from build123d import *

# Parameters (mm, degrees)
F0_W      = 38.3
F0_H      = 50.3
F0_W_2    = 28.3
F0_H_2    = 40.3
F4_DEPTH  = 4
F5_DEPTH  = 3
F5_FACE_W = 38.3
F5_FACE_H = 50.3
F7_DEPTH  = 35
F9_DEPTH  = 8
F10_R     = 5
F11_R     = 5


# Not quite as in the source:
# - the arcs of a loft's sections are written as splines that run evenly, so that the points pair up as in the source's solid


with BuildPart() as f4:
    # F0 (on Top) → F4 (new body)
    with BuildSketch(Plane.XY):
        Rectangle(F0_W, F0_H)
        Rectangle(F0_W_2, F0_H_2, mode=Mode.SUBTRACT)
    extrude(amount=-F4_DEPTH)

    # F0 (on Top) → F5 (join)
    with BuildSketch(Plane.XY):
        Rectangle(F0_W, F0_H)
        Rectangle(F0_W_2, F0_H_2, mode=Mode.SUBTRACT)
        Rectangle(F0_W_2, F0_H_2)
    extrude(amount=F5_DEPTH)

    # F5_face (on face) → F6 section 0
    with BuildSketch(Plane.XY.offset(3)):
        Rectangle(F5_FACE_W, F5_FACE_H)
    # F2 (on offset) → F6 section 1
    with BuildSketch(Plane.XY.offset(10)):
        with BuildLine():
            add(Edge.make_bspline(
                [(5.1493417049, 6.762712474), (4.2641047121, 7.436759727), (3.2451924408, 7.934526467), (1.09359433, 8.5024723272), (-0.0382449475, 8.5724279849), (-2.2434058754, 8.2737605906), (-3.3158598892, 7.9052550514), (-5.2388678728, 6.785443806), (-6.0886652211, 6.0345786977), (-6.762712474, 5.1493417049)],
                knots=[0, 0, 0, 0, 0.25, 0.25, 0.5, 0.5, 0.75, 0.75, 1, 1, 1, 1], degree=3))
            add(Edge.make_bspline(
                [(-6.762712474, 5.1493417049), (-7.436759727, 4.2641047121), (-7.934526467, 3.2451924408), (-8.5024723272, 1.09359433), (-8.5724279849, -0.0382449475), (-8.2737605906, -2.2434058754), (-7.9052550514, -3.3158598892), (-6.785443806, -5.2388678728), (-6.0345786977, -6.0886652211), (-5.1493417049, -6.762712474)],
                knots=[0, 0, 0, 0, 0.25, 0.25, 0.5, 0.5, 0.75, 0.75, 1, 1, 1, 1], degree=3))
            add(Edge.make_bspline(
                [(-5.1493417049, -6.762712474), (-4.2641047121, -7.436759727), (-3.2451924408, -7.934526467), (-1.09359433, -8.5024723272), (0.0382449475, -8.5724279849), (2.2434058754, -8.2737605906), (3.3158598892, -7.9052550514), (5.2388678728, -6.785443806), (6.0886652211, -6.0345786977), (6.762712474, -5.1493417049)],
                knots=[0, 0, 0, 0, 0.25, 0.25, 0.5, 0.5, 0.75, 0.75, 1, 1, 1, 1], degree=3))
            add(Edge.make_bspline(
                [(6.762712474, -5.1493417049), (7.436759727, -4.2641047121), (7.934526467, -3.2451924408), (8.5024723272, -1.09359433), (8.5724279849, 0.0382449475), (8.2737605906, 2.2434058754), (7.9052550514, 3.3158598892), (6.785443806, 5.2388678728), (6.0345786977, 6.0886652211), (5.1493417049, 6.762712474)],
                knots=[0, 0, 0, 0, 0.25, 0.25, 0.5, 0.5, 0.75, 0.75, 1, 1, 1, 1], degree=3))
        make_face()
    loft(ruled=True)

    # F7 (add): a face of the model
    f7_faces = [f4.faces().sort_by_distance(p)[0] for p in [
        (0, 0, 10),
    ]]
    extrude(f7_faces, amount=F7_DEPTH)

    # F3 (on Front) → F8 (revolve)
    with BuildSketch(Plane.XZ):
        with BuildLine():
            Line((0, 30.5), (0, 65.5))
            ThreePointArc((0, 65.5), (-12.3743686708, 60.3743686708), (-17.5, 48))
            Line((-17.5, 48), (0, 30.5))
        make_face()
        with BuildLine():
            ThreePointArc((-17.5, 48), (-12.3743686708, 60.3743686708), (0, 65.5))
            Line((0, 65.5), (-17.5, 65.5))
            Line((-17.5, 65.5), (-17.5, 48))
        make_face()
    revolve(axis=Axis((0, 0, 48), (0, 0, -1)))

    # F9 (cut): a face of the model
    f9_faces = [f4.faces().sort_by_distance(p)[0] for p in [
        (0, 0, 65.5),
    ]]
    extrude(f9_faces, amount=-F9_DEPTH, mode=Mode.SUBTRACT)

    # F10
    f10_edges = [f4.edges().sort_by_distance(p)[0] for p in [
        (17.5, 0, 57.5),
        (17.5, 0, 48),
    ]]
    fillet(f10_edges, radius=F10_R)

    # F11
    f11_edges = [f4.edges().sort_by_distance(p)[0] for p in [
        (-19.15, -25.15, -0.5),
        (-19.15, 25.15, -0.5),
        (19.15, 25.15, -0.5),
        (19.15, -25.15, -0.5),
    ]]
    fillet(f11_edges, radius=F11_R)


solid = f4.part
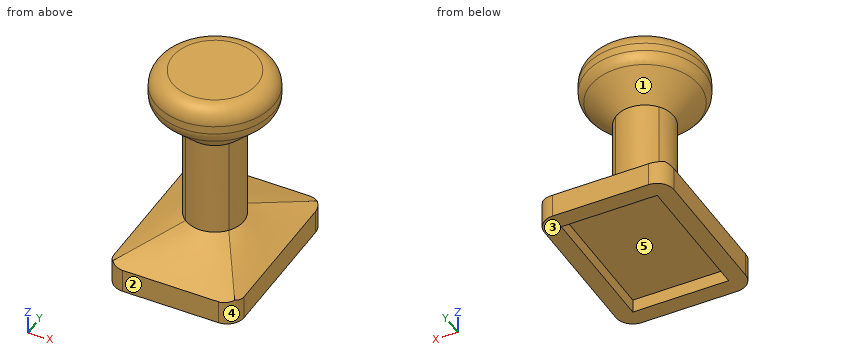
Check sheet for the modelled part. Datum: model origin and axes. Units: mm. Face numbers are marked on the shaded views. A direction names the side the tool comes from. Round coordinates to 2 decimals unless told otherwise and drop trailing zeros. Order: outer loops, then holes, each group sorted by start corner. A loop starts at its lowest first (then second) coordinate and runs counter-clockwise, first axis right, second up.
(1) Scan lines: probe 1 along Y at (x, z) = (-8.5, -0.5); probe 2 along Z at (x, y) = (6.5, 12.5); probe 3 along Z at (x, y) = (9, 14). Record each from-to range of solid material in increasing order.
(2) Go/stop test with flat-tipped pins: P1, Ø1, axis at x = -2.5, z = 33, coming from the -Y side; P2, Ø1.5, axis at x = -4, z = 16.5, coming from the -Y side; P3, Ø12, axis at x = -15, z = 44, coming from the +Y side. Record where each tip stops, or that it passes through.
(3) Cross-section at A-A, the plane z = 40. Enter the section's corners in (x, y), and give its area (3 significant figures).
(4) Access from +Z, -Z, +X, -X, +Y, -Y to the whole of each face (thin tool, end or side, straight path). Record for the marked faces 1 and 2.
(5) Draft check along Y on the marked faces 3, 4 and 5. Enter one of: pulls with the +Y half, pulls with the -Y half, needs draft (parallel to the pull), parting line crosses it, or undercut.
Check sheet entries:
1. probe 1: y = -25.15 to -20.15, 20.15 to 25.15
1. probe 2: z = 0 to 8.07, 44.59 to 57.24
1. probe 3: z = 0 to 7.36, 47.27 to 55.3
2. P1: stops at y = -8.26
2. P2: stops at y = -7.85
2. P3: stops at y = 13.42
3. outline: circle Ø19 at (0, 0)
3. area: 284 mm2
4. face 1: none
4. face 2: +Z, -Z, +X, -X, -Y
5. face 3: needs draft
5. face 4: pulls with the -Y half
5. face 5: undercut
